Design review of the part shown in the three views and the two pictorial views. Dimensions are in mm from the part's minimum x, y and z. A direction names the side the tool comes from. Coordinates: 2 decimals unless noted, no trailing zeros. Loops run counter-clockwise (first coordinate to the right, second up) from the corner with the lowest first, then second, coordinate; pieces in that order, holes last. Notation, with made-up numbers: (-38, 2) -> (-17, 2) arc R22 cw to (-17, 31) -> close; hole circle Ø4 at (40.5, 17.5). An arc over 180 degrees is marked (long way). Answer in a Markdown table with one row per item.
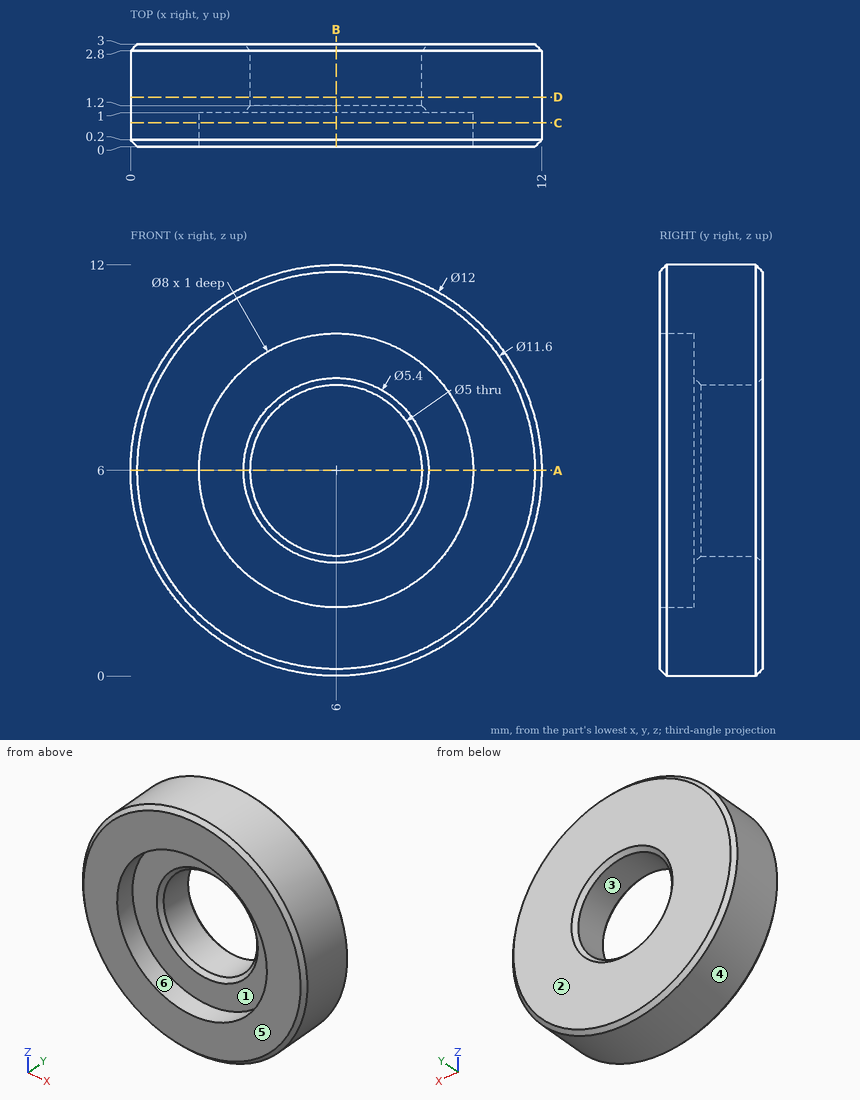
(1) Draft analysis for pull direction X (two halves, no side actions). For the marked faces 3, 4, 5 and 6, state which applies: pulls with the +X half, pulls with the -X half, needs draft (parallel to the pull), parting line crosses it, or undercut.
Evaluation:
| item | result |
|---|---|
| face 3 | undercut |
| face 4 | parting line crosses it |
| face 5 | needs draft |
| face 6 | undercut |
(2) Take a section at A-A on z = 6. Give the boundary of the cut face in (x, y).
Evaluation:
| item | result |
|---|---|
| outline | (0, 0.2) -> (0.2, 0) -> (2, 0) -> (2, 1) -> (3.3, 1) -> (3.5, 1.2) -> (3.5, 2.8) -> (3.3, 3) -> (0.2, 3) -> (0, 2.8) -> close; (8.5, 1.2) -> (8.7, 1) -> (10, 1) -> (10, 0) -> (11.8, 0) -> (12, 0.2) -> (12, 2.8) -> (11.8, 3) -> (8.7, 3) -> (8.5, 2.8) -> close |
(3) To check wall thickness, follow probe 1 along X at (y, z) = (2, 6); probe 2 along Z at (x, y) = (7, 2.2); probe 3 along Y at (x, z) = (7, 9.25). State the ranges of each line that lie inside material, in increasing order.
Evaluation:
| item | result |
|---|---|
| probe 1 | x = 0 to 3.5, 8.5 to 12 |
| probe 2 | z = 0.08 to 3.71, 8.29 to 11.92 |
| probe 3 | y = 1 to 3 |
(4) Take a section at B-B on x = 6. Give the boundary of the cut face in (y, z).
Evaluation:
| item | result |
|---|---|
| outline | (0, 0.2) -> (0.2, 0) -> (2.8, 0) -> (3, 0.2) -> (3, 3.3) -> (2.8, 3.5) -> (1.2, 3.5) -> (1, 3.3) -> (1, 2) -> (0, 2) -> close; (0, 10) -> (1, 10) -> (1, 8.7) -> (1.2, 8.5) -> (2.8, 8.5) -> (3, 8.7) -> (3, 11.8) -> (2.8, 12) -> (0.2, 12) -> (0, 11.8) -> close |
(5) Tool access review of the marked faces 1 and 2: name each direction out of +Z, -Z, +X, -X, +Y, -Y from which nothing blocks a thin tool from reaching the whole face with its end or side.
Evaluation:
| item | result |
|---|---|
| face 1 | -Y |
| face 2 | +Z, -Z, +X, -X, +Y |
(6) Take a section at D-D on y = 1.45. Give the boundary of the cut face in (x, z), and give its area (3 significant figures).
Evaluation:
| item | result |
|---|---|
| outline | circle Ø12 at (6, 6); hole circle Ø5 at (6, 6) |
| area | 93.5 mm² |
(7) Take a section at C-C on y = 0.7. Give the boundary of the cut face in (x, z).
Evaluation:
| item | result |
|---|---|
| outline | circle Ø12 at (6, 6); hole circle Ø8 at (6, 6) |
(8) For pin 1 (1 mm diameter, centred on x = 9.5, y = 2, fed in from -Z); pin 2 (4 mm diameter, centred on x = 6, z = 6, fed in from +Y); pin 3 (6.5 mm diameter, centred on x = 6, z = 6, fed in from -Y); pin 4 (1 mm diameter, centred on x = 3.5, y = 0.5, fed in from +Z), all flat-tipped, find the tip position at first contact; note any pin that passes through.
Evaluation:
| item | result |
|---|---|
| pin 1 | stops at z = 0.8 |
| pin 2 | passes through |
| pin 3 | stops at y = 1 |
| pin 4 | stops at z = 11.66 |
